The model under review builds one solid part; all positions refer to its coordinate system, in mm. Face numbers are marked on the shaded views. A direction names the side the tool comes from. Give positions to 0.01 mm unless a question says otherwise; leave off trailing zeros. Order: outer loops, then holes, each group sorted by start corner. A loop starts at its lowest first (then second) coordinate and runs counter-clockwise, first axis right, second up. Notation, with made-up numbers: (-11, 4) - (44, 4) arc R32 cw to (44, 30) - close; hole circle Ø1 at (44.5, 2.25). An arc over 180 degrees is marked (long way). Put each result on its own line as item: value.
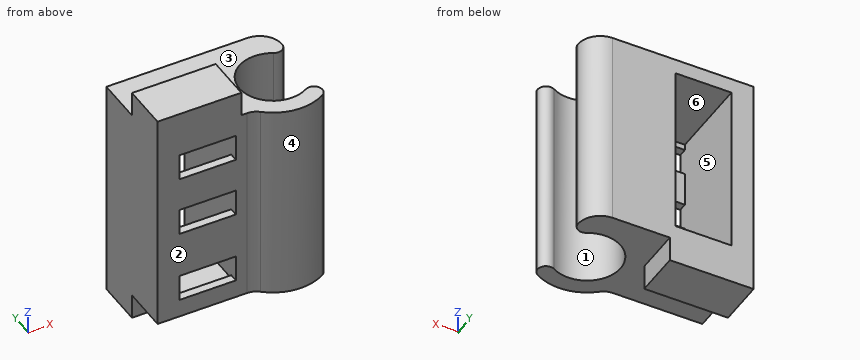
Autodesk Inventor part; units mm, degrees
ref_plane "YZ Plane" through (0, 0, 0) normal (1, 0, 0) x (0, 1, 0)
ref_plane "XZ Plane" through (0, 0, 0) normal (0, 1, 0) x (-1, 0, 0)
ref_plane "XY Plane" through (0, 0, 0) normal (0, 0, 1) x (1, 0, 0)
sketch "Sketch1" plane through (0, 0, 0) normal (0, 0, 1) x (1, 0, 0)
  line L0 (-6, 5.5) -> (6, 5.5)
  line L1 (6, 5.5) -> (6, -5.5)
  line L2 (6, -5.5) -> (-6, -5.5)
  line L3 (-6, -5.5) -> (-6, 5.5)
  point P0 (0, 0)
  point P1 (6, 0)
  point P2 (0, 5.5)
  dimension "d0" = 12
  dimension "d1" = 11
extrude "Extrusion1" add sketch "Sketch1" along normal blind 24
sketch "Sketch2" plane through (-6, 5.5, 0) normal (0, 1, 0) x (1, 0, 0)
  line L0 (2.65, -22.2) -> (9.35, -22.2)
  line L1 (9.35, -22.2) -> (9.35, -1.8)
  line L2 (9.35, -1.8) -> (2.65, -1.8)
  line L3 (2.65, -1.8) -> (2.65, -22.2)
  line L4 (0, 0) -> (0, -24)
  line L5 (0, 0) -> (12, 0)
  point P0 (6, 0)
  point P1 (2.65, -12)
  point P2 (0, -12)
  point P3 (6, -1.8)
  point P4 (6, 0)
  dimension "d4" = 20.4
  dimension "d5" = 6.7
extrude "Extrusion2" cut sketch "Sketch2" against normal blind 10
sketch "Sketch3" plane through (-6, -4.5, 0) normal (0, 1, 0) x (1, 0, 0)
  line L0 (2.65, -22.2) -> (2.65, -1.8)
  line L1 (9.35, -1.8) -> (9.35, -22.2)
  line L2 (2.65, -21.5) -> (9.35, -21.5)
  line L3 (9.35, -21.5) -> (9.35, -18.3)
  line L4 (9.35, -18.3) -> (2.65, -18.3)
  line L5 (2.65, -18.3) -> (2.65, -21.5)
  line L6 (2.65, -14.2) -> (9.35, -14.2)
  line L7 (9.35, -14.2) -> (9.35, -11)
  line L8 (9.35, -11) -> (2.65, -11)
  line L9 (2.65, -11) -> (2.65, -14.2)
  line L10 (2.65, -5.4) -> (9.35, -5.4)
  line L11 (9.35, -5.4) -> (9.35, -2.2)
  line L12 (9.35, -2.2) -> (2.65, -2.2)
  line L13 (2.65, -2.2) -> (2.65, -5.4)
  line L14 (9.35, -22.2) -> (2.65, -22.2)
  line L15 (2.65, -1.8) -> (9.35, -1.8)
  point P0 (6, 0)
  point P1 (2.65, -19.9)
  point P2 (2.65, -12.6)
  point P3 (2.65, -3.8)
  dimension "d9" = 7.3
  dimension "d10" = 8.8
  dimension "d11" = 3.2
  dimension "d12" = 3.2
  dimension "d13" = 3.2
  dimension "d39" = 2
extrude "Extrusion3" cut sketch "Sketch3" against normal blind 10 contours L0 L4 L1 L2 | L0 L8 L1 L6 | L0 L12 L1 L10
sketch "Sketch4" plane through (0, 0, 24) normal (0, 0, 1) x (1, 0, 0)
  line L0 (6, 5.5) -> (-6, 5.5)
  circle A0 centre (10, -1.5) radius 4
  arc A1 (6, 2.9721) -> (13, -6.6962) centre (10, -1.5) ccw
  arc A2 (12, 1.9641) -> (13.5, 2.8301) centre (12.5, 2.8301) ccw
  arc A3 (13, -6.6962) -> (12, -4.9641) centre (12.5, -5.8301) ccw
  line L1 (6, -5.5) -> (6, 5.5)
  line L2 (6, 2.9721) -> (6, -5.9721)
  circle A4 centre (10, -1.5) radius 4
  arc A5 (6, 2.9721) -> (13, -6.6962) centre (10, -1.5) ccw
  line L3 (6, 5.5) -> (10.8301, 5.5)
  line L4 (6, 5.5) -> (6, 2.9721)
  arc A6 (13.5, 2.8301) -> (10.8301, 5.5) centre (10.8301, 2.8301) ccw
  point P0 (0, 0)
  dimension "d31" = 8
  dimension "d32" = 12
  dimension "d33" = 7
  dimension "d34" = 2.5
extrude "Extrusion4" add sketch "Sketch4" against normal blind 24 contours A0 L1 L3 A6 A2 | A3 A1 L2 L1 A0 | L1 L2 A1
sketch "Sketch5" plane through (0, 0, 0) normal (0, 0, -1) x (-1, 0, 0)
  line L0 (6, 5.5) -> (-6, 5.5)
  line L1 (6, 5.5) -> (-4, 5.5)
  line L2 (-4, 5.5) -> (-4, 0)
  line L3 (-4, 0) -> (6, 0)
  line L4 (6, 0) -> (6, 5.5)
  dimension "d35" = 10
  dimension "d36" = 5.5
extrude "Extrusion5" add sketch "Sketch5" along normal blind 3
sketch "Sketch6" plane through (0, 0, 24) normal (0, 0, 1) x (1, 0, 0)
  line L0 (-6, -5.5) -> (-6, 0)
  line L1 (-6, -5.5) -> (4, -5.5)
  line L2 (4, -5.5) -> (4, 0)
  line L3 (4, 0) -> (-6, 0)
  line L4 (-6, 0) -> (-6, -5.5)
  dimension "d37" = 10
  dimension "d38" = 5.5
extrude "Extrusion6" add sketch "Sketch6" along normal blind 3
fillet "Fillet2" radius 2 1 edges at (5.5279, -5.5, 12)
properties part number "Switch holder_Right"
(1) For the marked faces 1 and 2, list the 3-axis set-ups (+Z, -Z, +X, -X, +Y, -Y) from which the entire face can be reached by the end or side of a thin tool; tool diameter is ignored.
The answers:
face 1: +Z, -Z
face 2: +Z, -Z, -X, -Y
(2) Wall thickness on L1, parallel to Y at x = 10, z = 16.75; L2, parallel to Z at x = 0.5, y = 3.5; L3, parallel to X at y = -1.5, z = 13.75: over which ranges is each line inside the solid? List them lowest first.
The answers:
L1: -7.5 to -5.5, 2.5 to 5.5
L2: -3 to 1.8, 22.2 to 24
L3: -6 to -3.35, 3.35 to 6
(3) The part is to be moulded in two halves that separate along X. For the marked faces 3, 4, 5 and 6, say which applies: pulls with the +X half, pulls with the -X half, needs draft (parallel to the pull), parting line crosses it, or undercut.
The answers:
face 3: needs draft
face 4: parting line crosses it
face 5: undercut
face 6: undercut
(4) Take a section at A-A, the plane x = 10. Write out the cut boundary in (y, z), then the cut area to 3 significant figures.
The answers:
outline: (-7.5, 0) - (-5.5, 0) - (-5.5, 24) - (-7.5, 24) - close; (2.5, 0) - (5.5, 0) - (5.5, 24) - (2.5, 24) - close
area: 120 mm^2
(5) Take a section at B-B, the plane x = -0.75. Write out the cut boundary in (y, z), then the cut area to 3 significant figures.
The answers:
outline: (-5.5, 0) - (0, 0) - (0, -3) - (5.5, -3) - (5.5, 1.8) - (-4.5, 1.8) - (-4.5, 2.2) - (-5.5, 2.2) - close; (-5.5, 5.4) - (-4.5, 5.4) - (-4.5, 11) - (-5.5, 11) - close; (-5.5, 14.2) - (-4.5, 14.2) - (-4.5, 18.3) - (-5.5, 18.3) - close; (-5.5, 21.5) - (-4.5, 21.5) - (-4.5, 22.2) - (5.5, 22.2) - (5.5, 24) - (0, 24) - (0, 27) - (-5.5, 27) - close
area: 83.4 mm^2
(6) Take a section at C-C, the plane y = -1.5. Write out the cut boundary in (x, z), then the cut area to 3 significant figures.
The answers:
outline: (-6, 0) - (6, 0) - (6, 24) - (4, 24) - (4, 27) - (-6, 27) - close; hole (-3.35, 1.8) - (3.35, 1.8) - (3.35, 22.2) - (-3.35, 22.2) - close
area: 181 mm^2
(7) Take a section at D-D, the plane z = 4.5. Write out the cut boundary in (x, y), then the cut area to 3 significant figures.
The answers:
outline: (-6, -5.5) - (-3.35, -5.5) - (-3.35, 5.5) - (-6, 5.5) - close; (3.35, -5.5) - (4.71, -5.5) arc R2 cw to (6.03, -6) arc R6 ccw to (13, -6.7) arc R1 ccw to (12, -4.96) arc R4 cw (long way) to (12, 1.96) arc R1 ccw to (13.5, 2.83) arc R2.67 ccw to (10.83, 5.5) - (3.35, 5.5) - close
area: 100 mm^2
(8) Clearance check with flat-ended pins moving along their axes: pin 1 Ø5 at (x, z) = (6.5, 10.5) entering from -Y; pin 2 Ø1 at (x, y) = (4.5, 2.5) entering from +Z; pin 3 Ø6 at (y, z) = (-2, 4.5) entering from +X. State where each tip first meets the part, or that it passes through.
The answers:
pin 1: y = -7.42
pin 2: z = 24
pin 3: x = 13.06
